The model under review builds one solid part; all positions refer to its coordinate system, in mm. Face numbers are marked on the shaded views. A direction names the side the tool comes from. Coordinates: 2 decimals unless noted, no trailing zeros. Write each loop counter-clockwise with the first axis right and the second up, starting at its lowest first coordinate (ties: lowest second). Pieces come first, ordered by that corner, then holes. Notation, with made-up numbers: (9, 75.25) - (27, 75.25) arc R12 cw to (27, 89.25) - close; hole circle Ø10 at (-6, 27). An arc over 180 degrees is marked (long way). Put each result on its own line as item: value.
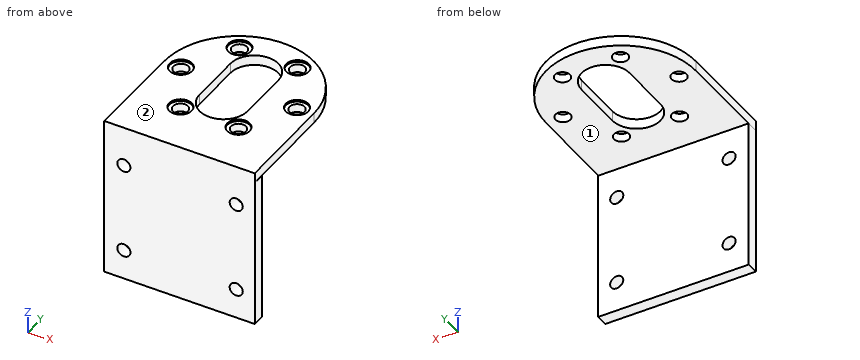
from build123d import *

# Parameters (mm, degrees)
SKETCH_1_W          = 40.2
SKETCH_1_H          = 43
EXTRUDE_1_DEPTH     = 3.2
SKETCH_3_W          = 40.2
SKETCH_3_H          = 2.7
EXTRUDE_3_DEPTH     = 43.8
SKETCH_4_OUTSIDE_W  = 57.266
SKETCH_4_OUTSIDE_H  = 64.066
CUT_EXTRUDE_2_DEPTH = 2.7
SKETCH_5_R          = 1.75
CUT_EXTRUDE_3_DEPTH = 53.770256774
CUT_EXTRUDE_4_DEPTH = 3.2
SKETCH_7_R          = 2
CUT_EXTRUDE_5_DEPTH = 3.2
SKETCH_8_R          = 3
CUT_EXTRUDE_6_DEPTH = 0.5


with BuildPart() as part:
    # 草图1 → 凸台-拉伸1 (new body)
    with BuildSketch(Plane(origin=(0, 0, 0), x_dir=(1, 0, 0), z_dir=(0, 1, 0))):
        Rectangle(SKETCH_1_W, SKETCH_1_H)
    extrude(amount=EXTRUDE_1_DEPTH)

    # 草图3 → 凸台-拉伸3 (add)
    with BuildSketch(Plane(origin=(0, 3.2, 0), x_dir=(1, 0, 0), z_dir=(0, 1, 0))):
        with Locations((0, -20.15)):
            Rectangle(SKETCH_3_W, SKETCH_3_H)
    extrude(amount=EXTRUDE_3_DEPTH)

    # 草图4 outside → 切除-拉伸2 (cut)
    with BuildSketch(Plane.XY.offset(21.5)):
        with Locations((0, 23.5)):
            Rectangle(SKETCH_4_OUTSIDE_W, SKETCH_4_OUTSIDE_H)
        with BuildLine():
            Line((-20, 27), (-20.1, 0))
            Line((-20.1, 0), (20.1, 0))
            Line((20.1, 0), (20, 27))
            ThreePointArc((20, 27), (0, 47), (-20, 27))
        make_face(mode=Mode.SUBTRACT)
    extrude(amount=-CUT_EXTRUDE_2_DEPTH, mode=Mode.SUBTRACT)

    # 草图5 → 切除-拉伸3 (cut, through all)
    with BuildSketch(Plane(origin=(0, 3.2, 0), x_dir=(1, 0, 0), z_dir=(0, 1, 0))):
        with Locations(Location((-14.85, 13.45, 0), (0, 0, 270))):
            Circle(SKETCH_5_R)
        with Locations(Location((15.15, -10.75, 0), (0, 0, 270))):
            Circle(SKETCH_5_R)
        with Locations(Location((-14.85, -10.75, 0), (0, 0, 270))):
            Circle(SKETCH_5_R)
        with Locations(Location((15.15, 13.45, 0), (0, 0, 270))):
            Circle(SKETCH_5_R)
    extrude(amount=-CUT_EXTRUDE_3_DEPTH, mode=Mode.SUBTRACT)

    # 草图6 → 切除-拉伸4 (cut)
    with BuildSketch(Plane.XY.offset(21.5)):
        with BuildLine():
            Line((-6.4, 34), (-6.4, 20))
            ThreePointArc((-6.4, 20), (0, 13.6), (6.4, 20))
            Line((6.4, 20), (6.4, 34))
            ThreePointArc((6.4, 34), (0, 40.4), (-6.4, 34))
        make_face()
    extrude(amount=-CUT_EXTRUDE_4_DEPTH, mode=Mode.SUBTRACT)

    # 草图7 → 切除-拉伸5 (cut)
    with BuildSketch(Plane.XY.offset(21.5)):
        with Locations((-7.75, 40.4)):
            Circle(SKETCH_7_R)
        with Locations((7.75, 40.4)):
            Circle(SKETCH_7_R)
        with Locations((-15.5, 27)):
            Circle(SKETCH_7_R)
        with Locations((15.5, 27)):
            Circle(SKETCH_7_R)
        with Locations((-7.75, 13.6)):
            Circle(SKETCH_7_R)
        with Locations((7.75, 13.6)):
            Circle(SKETCH_7_R)
    extrude(amount=-CUT_EXTRUDE_5_DEPTH, mode=Mode.SUBTRACT)

    # 草图8 → 切除-拉伸6 (cut)
    with BuildSketch(Plane.XY.offset(21.5)):
        with Locations((-7.75, 40.4)):
            Circle(SKETCH_8_R)
        with Locations((7.75, 40.4)):
            Circle(SKETCH_8_R)
        with Locations((-15.5, 27)):
            Circle(SKETCH_8_R)
        with Locations((15.5, 27)):
            Circle(SKETCH_8_R)
        with Locations((-7.75, 13.6)):
            Circle(SKETCH_8_R)
        with Locations((7.75, 13.6)):
            Circle(SKETCH_8_R)
    extrude(amount=-CUT_EXTRUDE_6_DEPTH, mode=Mode.SUBTRACT)


solid = part.part
1. To check wall thickness, follow probe 1 along Y at (x, z) = (7.75, 20.5); probe 2 along Y at (x, z) = (-7.75, 21.15); probe 3 along Y at (x, z) = (14, 6). State the ranges of each line that lie inside material, in increasing order.
Determined:
probe 1: y = 0 to 11.6, 15.6 to 38.4, 42.4 to 45.44
probe 2: y = 0 to 10.6, 16.6 to 37.4, 43.4 to 45.44
probe 3: y = 0 to 3.2
2. Consider section A-A on z = -13.45. State the section outline as (x, y) points, plus the area to 3 significant figures.
Determined:
outline: (-20.1, 0) - (-16.6, 0) - (-16.6, 3.2) - (-20.1, 3.2) - close; (-13.1, 0) - (13.4, 0) - (13.4, 3.2) - (-13.1, 3.2) - close; (16.9, 0) - (20.1, 0) - (20.1, 3.2) - (16.9, 3.2) - close
area: 106 mm^2
3. Consider section D-D on x = -14.85. State the section outline as (y, z) points.
Determined:
outline: (0, -21.5) - (3.2, -21.5) - (3.2, -15.2) - (0, -15.2) - close; (0, -11.7) - (3.2, -11.7) - (3.2, 9) - (0, 9) - close; (0, 12.5) - (3.2, 12.5) - (3.2, 18.8) - (25.11, 18.8) - (25.11, 21) - (24.07, 21) - (24.07, 21.5) - (0, 21.5) - close; (28.89, 18.8) - (40.4, 18.8) - (40.4, 21.5) - (29.93, 21.5) - (29.93, 21) - (28.89, 21) - close
4. Consider section B-B on z = 19.5. State the section outline as (x, y) points, plus the area to 3 significant figures.
Determined:
outline: (-20.1, 0) - (20.1, 0) - (20, 27) arc R20 ccw to (-20, 27) - close; hole circle Ø4 at (-15.5, 27); hole circle Ø4 at (-7.75, 13.6); hole circle Ø4 at (-7.75, 40.4); hole (-6.4, 20) arc R6.4 ccw to (6.4, 20) - (6.4, 34) arc R6.4 ccw to (-6.4, 34) - close; hole circle Ø4 at (7.75, 13.6); hole circle Ø4 at (7.75, 40.4); hole circle Ø4 at (15.5, 27)
area: 1,330 mm^2
5. For pin 1 Ø5.5 at (x, z) = (15.15, 10.75) entering from +Y; pin 2 Ø9.5 at (x, y) = (7.75, 40.4) entering from -Z; pin 3 Ø9.5 at (x, y) = (15.5, 27) entering from +Z, all flat-tipped, find the tip position at first contact; note any pin that passes through.
Determined:
pin 1: stops at y = 3.2
pin 2: stops at z = 18.8
pin 3: stops at z = 21.5
6. Consider section C-C on x = -7.75. State the section outline as (y, z) points, plus the area to 3 significant figures.
Determined:
outline: (0, -21.5) - (3.2, -21.5) - (3.2, 18.8) - (11.6, 18.8) - (11.6, 21) - (10.6, 21) - (10.6, 21.5) - (0, 21.5) - close; (15.6, 18.8) - (38.4, 18.8) - (38.4, 21) - (37.4, 21) - (37.4, 21.5) - (16.6, 21.5) - (16.6, 21) - (15.6, 21) - close; (42.4, 18.8) - (45.44, 18.8) - (45.44, 21.5) - (43.4, 21.5) - (43.4, 21) - (42.4, 21) - close
area: 228 mm^2
7. Machinability: for the marked faces 1 and 2, which of the approach directions +Z, -Z, +X, -X, +Y, -Y give a long, thin tool a straight path to every point of the face, cutting with its end or side? Answer none if there is none.
Determined:
face 1: -Z, +X, -X, +Y
face 2: +Z, +X, -X, +Y, -Y
